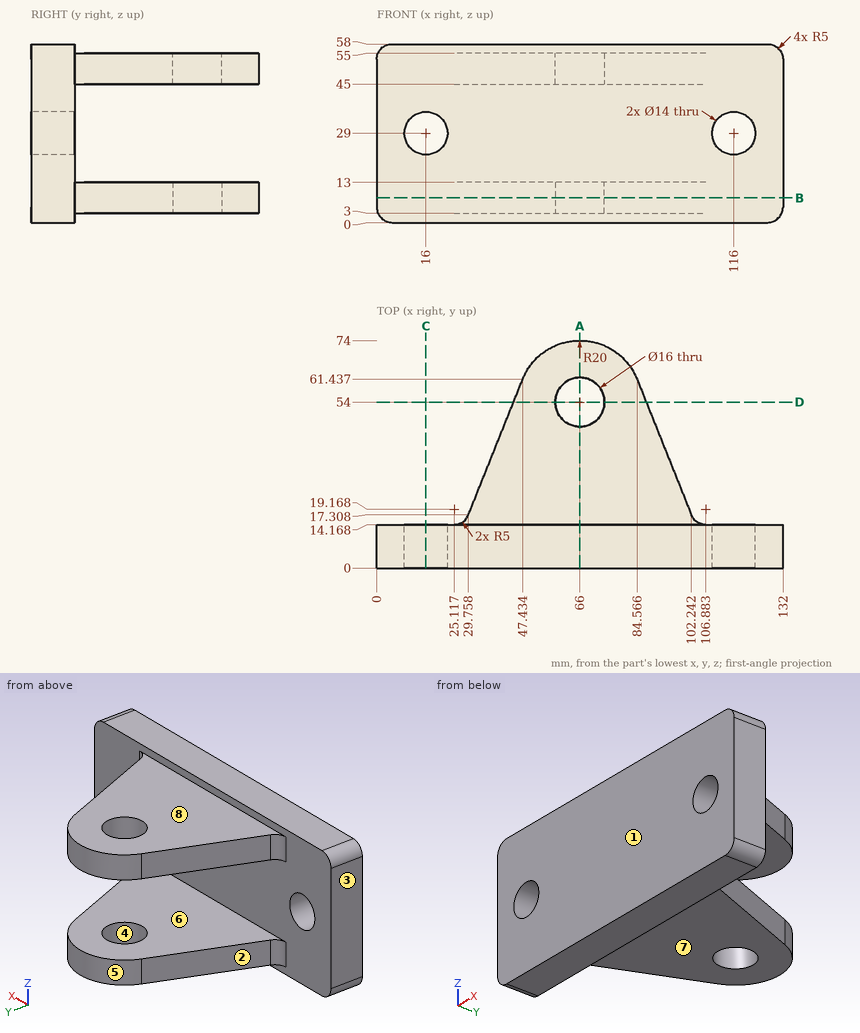
Input: dimensioned drawing with shaded views. Units: mm. Origin: part minimum x, y, z. A direction names the side the tool comes from. Round coordinates to 2 decimals unless told otherwise and drop trailing zeros. Order: outer loops, then holes, each group sorted by start corner. A loop starts at its lowest first (then second) coordinate and runs counter-clockwise, first axis right, second up. Notation, with made-up numbers: (-1.75, -0.75) -> (14.25, -0.75) arc R23 ccw to (14.25, 37.25) -> close; hole circle Ø8 at (-12, 15.25). An arc over 180 degrees is marked (long way). One line per item, written item: value. Start each with the question number.
Q1. Section query D-D (y = 54). Return the cut outline in (x, z) (1 decimal), plus the area to 3 significant figures.
Q2. Access query for the marked faces 5, 6, 7 and 8. Directions: +Z, -Z, +X, -X, +Y, -Y. A direction counts if a zero-diameter tool reaches every point of the face in a straight line with its end or side. Return the directions, or none.
Q3. Section query B-B (z = 8). Return the cut outline in (x, y).
Q4. Section query C-C (x = 16). Return the cut outline in (y, z).
Q5. Section query A-A (x = 66). Return the cut outline in (y, z).
Q6. Pin query (flat end, axial travel): pin 1 (5 mm diameter, centred on x = 40.5, y = 52, fed in from +Z); pin 2 (2 mm diameter, centred on x = 31.5, y = 20.5, fed in from -Z); pin 3 (18.5 mm diameter, centred on x = 66, y = 54, fed in from +Z); pin 4 (12 mm diameter, centred on x = 43.5, z = 26, fed in from +Y). Return the tip coordinate at first contact, or that it passes through.
Q7. Draft query along Y for the marked faces 1, 2, 3 and 4. Return one class per face: pulls with the +Y half, pulls with the -Y half, needs draft (parallel to the pull), parting line crosses it, or undercut.
Q8. Material intervals for probe 1 along X at (y, z) = (6.75, 29); probe 2 along Z at (x, y) = (38, 18.5); probe 3 along Z at (x, y) = (116, 6.5), sorted ascending.
Findings below:
1. outline: (44.5, 3) -> (58, 3) -> (58, 13) -> (44.5, 13) -> close; (44.5, 45) -> (58, 45) -> (58, 55) -> (44.5, 55) -> close; (74, 3) -> (87.5, 3) -> (87.5, 13) -> (74, 13) -> close; (74, 45) -> (87.5, 45) -> (87.5, 55) -> (74, 55) -> close
1. area: 542 mm²
2. face 5: +Z, -Z, +Y
2. face 6: +X, -X, +Y
2. face 7: -Z, +X, -X, +Y
2. face 8: +Z, +X, -X, +Y
3. outline: (0, 0) -> (132, 0) -> (132, 14.17) -> (106.88, 14.17) arc R5 cw to (102.24, 17.31) -> (84.57, 61.44) arc R20 ccw to (47.43, 61.44) -> (29.76, 17.31) arc R5 cw to (25.12, 14.17) -> (0, 14.17) -> close; hole circle Ø16 at (66, 54)
4. outline: (0, 0) -> (14.17, 0) -> (14.17, 22) -> (0, 22) -> close; (0, 36) -> (14.17, 36) -> (14.17, 58) -> (0, 58) -> close
5. outline: (0, 0) -> (14.17, 0) -> (14.17, 3) -> (46, 3) -> (46, 13) -> (14.17, 13) -> (14.17, 45) -> (46, 45) -> (46, 55) -> (14.17, 55) -> (14.17, 58) -> (0, 58) -> close; (62, 3) -> (74, 3) -> (74, 13) -> (62, 13) -> close; (62, 45) -> (74, 45) -> (74, 55) -> (62, 55) -> close
6. pin 1: through
6. pin 2: z = 3
6. pin 3: z = 55
6. pin 4: y = 14.17
7. face 1: pulls with the -Y half
7. face 2: pulls with the +Y half
7. face 3: needs draft
7. face 4: undercut
8. probe 1: 0 to 9, 23 to 109, 123 to 132
8. probe 2: 3 to 13, 45 to 55
8. probe 3: 0 to 22, 36 to 58
